Can you work these out from the drawing? Everything is in mm from the part's minimum corner. Coordinates: 2 decimals unless noted, no trailing zeros. Order: outer loops, then holes, each group sorted by start corner. A loop starts at its lowest first (then second) coordinate and runs counter-clockwise, first axis right, second up. Notation, with made-up numbers: M -12,40.25 L 2,40.25 A14 cw 2,51.25 Z; hole C -26.5,-38 d3. An arc over 180 degrees is marked long. One line per question, with ' | ' between items. Start each with the question number.
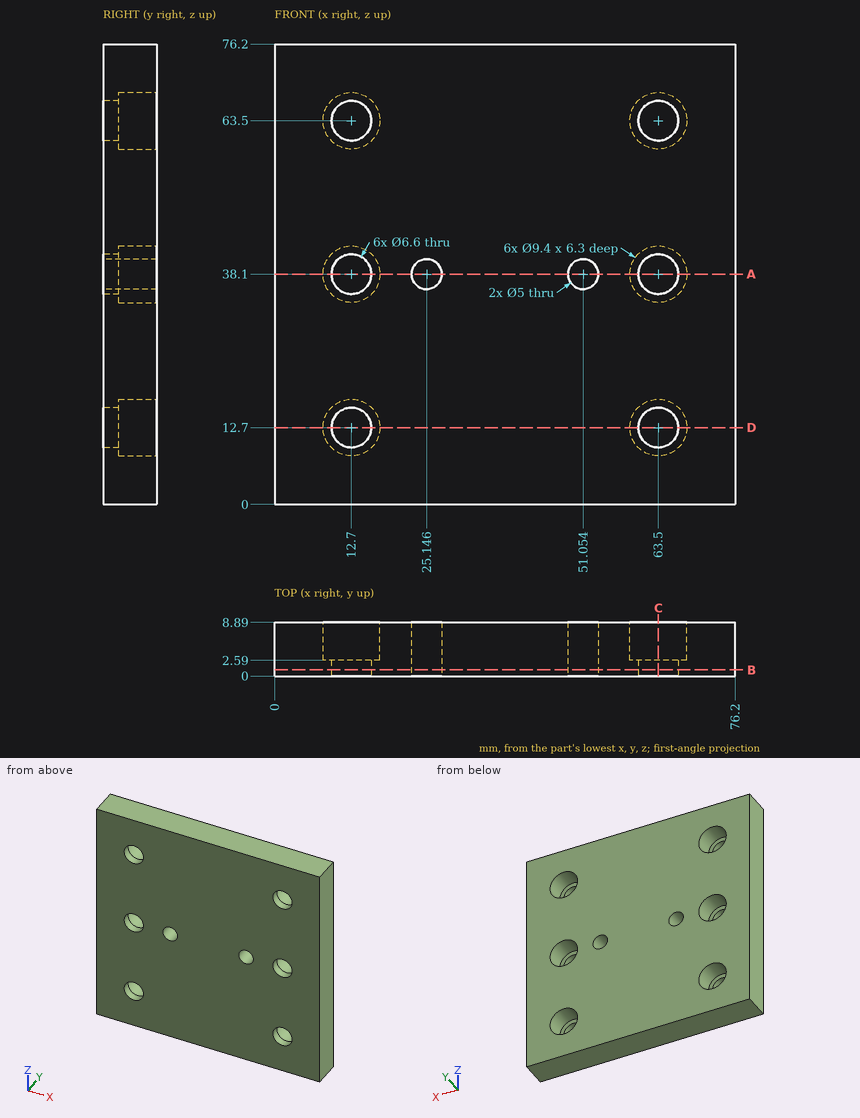
(1) For P1, Ø5.5, axis at x = 12.7, z = 63.5, coming from the +Y side; P2, Ø3, axis at x = 12.5, z = 40, coming from the +Y side, each with a flat end and sliding along its axis, tell me the tip position at first contact or that it passes through.
(2) Imagine slicing it at B-B, the plane y = 1. Count the separate pieces of the cut face and the enclosed holes in it, plus the area to 3 significant figures.
(3) Imagine slicing it at A-A, the plane z = 38.1. Write out the boundary of the cut face in (x, y), plus the area to 3 significant figures.
(4) If I drill on line 1 along X through (y, z) = (6.75, 38.1); line 2 along X through (y, z) = (1.4, 63.5); line 3 along Z through (x, y) = (63.5, 4.5), over which ranges is the centre line in solid material (lowest first)? Write a range as from..to.
(5) Imagine slicing it at D-D, the plane z = 12.7. Write out the boundary of the cut face in (x, y), plus the area to 3 significant figures.
(6) Imagine slicing it at C-C, the plane x = 63.5. Write out the boundary of the cut face in (y, z).
Answers:
1) P1: through | P2: y = 2.59
2) separate pieces: 1 | enclosed holes: 8 | area: 5,560 mm²
3) outline: M 0,0 L 9.4,0 L 9.4,2.59 L 8,2.59 L 8,8.89 L 0,8.89 Z; M 16,0 L 22.65,0 L 22.65,8.89 L 17.4,8.89 L 17.4,2.59 L 16,2.59 Z; M 27.65,0 L 48.55,0 L 48.55,8.89 L 27.65,8.89 Z; M 53.55,0 L 60.2,0 L 60.2,2.59 L 58.8,2.59 L 58.8,8.89 L 53.55,8.89 Z; M 66.8,0 L 76.2,0 L 76.2,8.89 L 68.2,8.89 L 68.2,2.59 L 66.8,2.59 Z | area: 436 mm²
4) line 1: 0..8, 17.4..22.65, 27.65..48.55, 53.55..58.8, 68.2..76.2 | line 2: 0..9.4, 16..60.2, 66.8..76.2 | line 3: 0..8, 17.4..33.4, 42.8..58.8, 68.2..76.2
5) outline: M 0,0 L 9.4,0 L 9.4,2.59 L 8,2.59 L 8,8.89 L 0,8.89 Z; M 16,0 L 60.2,0 L 60.2,2.59 L 58.8,2.59 L 58.8,8.89 L 17.4,8.89 L 17.4,2.59 L 16,2.59 Z; M 66.8,0 L 76.2,0 L 76.2,8.89 L 68.2,8.89 L 68.2,2.59 L 66.8,2.59 Z | area: 525 mm²
6) outline: M 0,0 L 8.89,0 L 8.89,8 L 2.59,8 L 2.59,9.4 L 0,9.4 Z; M 0,16 L 2.59,16 L 2.59,17.4 L 8.89,17.4 L 8.89,33.4 L 2.59,33.4 L 2.59,34.8 L 0,34.8 Z; M 0,41.4 L 2.59,41.4 L 2.59,42.8 L 8.89,42.8 L 8.89,58.8 L 2.59,58.8 L 2.59,60.2 L 0,60.2 Z; M 0,66.8 L 2.59,66.8 L 2.59,68.2 L 8.89,68.2 L 8.89,76.2 L 0,76.2 Z
